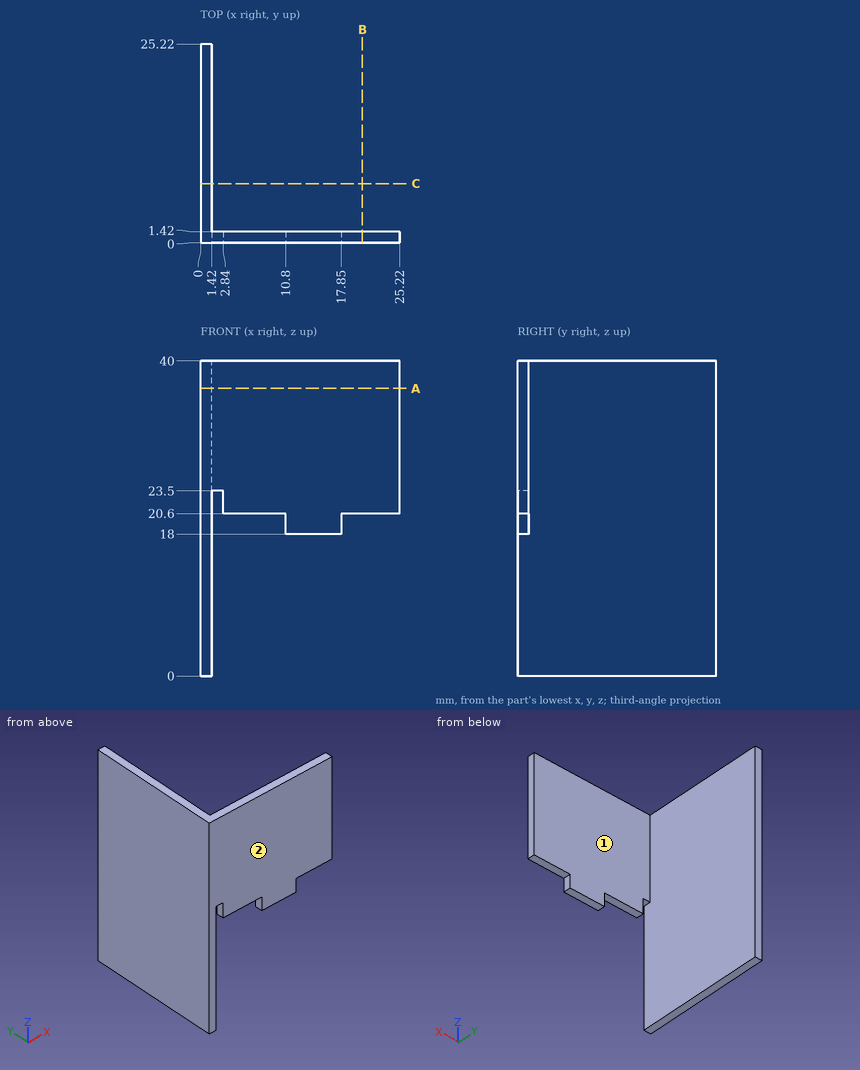
Geometry: see drawing. Coordinates: mm, zero at the bounding-box minimum. A direction names the side the tool comes from. Round coordinates to 2 decimals unless told otherwise and drop trailing zeros. Loops run counter-clockwise (first coordinate to the right, second up) from the corner with the lowest first, then second, coordinate; pieces in that order, holes last. Notation, with made-up numbers: M 76.25,-5.75 L 85.25,-5.75 A27 ccw 85.25,10.25 Z; hole C 69.5,14.25 d5. An arc over 180 degrees is marked long. Use a Markdown table: item, result. Add a question column.
1. Cut plane B-B, the plane x = 20.5. Output: boundary loops of the cut face in (y, z).
2. Cut plane A-A, the plane z = 36.5. Output: boundary loops of the cut face in (x, y).
3. Cut plane C-C, the plane y = 7.5. Output: boundary loops of the cut face in (x, z), and give its area (3 significant figures).
4. Contact query for flat-ended pins moving along their axis: pin 1 (1 mm diameter, centred on x = 21, z = 34, fed in from +Y); pin 2 (0.7 mm diameter, centred on x = 7, y = 1, fed in from -Z); pin 3 (0.7 mm diameter, centred on y = 0.5, z = 19, fed in from +X). Output: stop coordinate, or through.
5. Set-up query: the marked faces 1 and 2. Return all of +Z, -Z, +X, -X, +Y, -Y with unobstructed straight access to the full face (end or side cutting, diameter ignored); none if empty.
6. Ray query, line 1 along X through (y, z) = (17.25, 8). Return the intervals inside material, ascending. Write a range as [from, to].
Solution:
| question | item | result |
|---|---|---|
| 1 | outline | M 0,20.6 L 1.42,20.6 L 1.42,40 L 0,40 Z |
| 2 | outline | M 0,0 L 25.22,0 L 25.22,1.42 L 1.42,1.42 L 1.42,25.22 L 0,25.22 Z |
| 3 | outline | M 0,0 L 1.42,0 L 1.42,40 L 0,40 Z |
| 3 | area | 56.8 mm2 |
| 4 | pin 1 | stops at y = 1.42 |
| 4 | pin 2 | stops at z = 20.6 |
| 4 | pin 3 | stops at x = 17.85 |
| 5 | face 1 | +Z, -Z, +X, +Y |
| 5 | face 2 | +Z, -Z, +X, -X, -Y |
| 6 | line 1 | x = [0, 1.42] |
